Verification items for the finished model (mm, model axes). Coordinates: 2 decimals unless noted, no trailing zeros. Write each loop counter-clockwise with the first axis right and the second up, starting at its lowest first coordinate (ties: lowest second). Pieces come first, ordered by that corner, then holes. Notation, with made-up numbers: M -28,84 L 19,84 A22 ccw 19,102 Z; hole C -38.75,-0.5 d3. An arc over 180 degrees is marked long. Answer in a Markdown table with one row per item.
from build123d import *

# Parameters (mm, degrees)
SKETCH1_W           = 45
SKETCH1_H           = 75
BOSS_EXTRUDE1_DEPTH = 1
SKETCH2_W           = 23
SKETCH2_H           = 16.479286024
BOSS_EXTRUDE2_DEPTH = 1
SKETCH3_W           = 15.006040788
SKETCH3_H           = 6.122008564
BOSS_EXTRUDE3_DEPTH = 1


with BuildPart() as part:
    # Sketch1 → Boss-Extrude1 (new body)
    with BuildSketch(Plane.XY):
        Rectangle(SKETCH1_W, SKETCH1_H)
    extrude(amount=BOSS_EXTRUDE1_DEPTH)

    # Sketch2 → Boss-Extrude2 (add)
    with BuildSketch(Plane.XY.offset(1)):
        with Locations((11, -45.739643012)):
            Rectangle(SKETCH2_W, SKETCH2_H)
    extrude(amount=-BOSS_EXTRUDE2_DEPTH)

    # Sketch3 → Boss-Extrude3 (add)
    with BuildSketch(Plane.XY.offset(1)):
        with Locations((-14.996979606, 40.561004282)):
            Rectangle(SKETCH3_W, SKETCH3_H)
    extrude(amount=-BOSS_EXTRUDE3_DEPTH)


solid = part.part
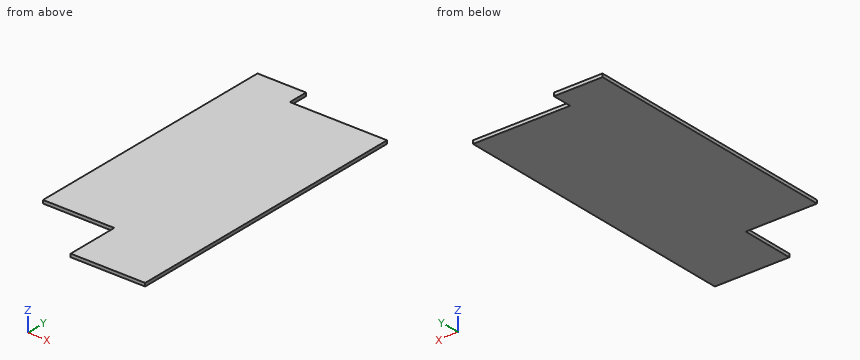
1) Depth check by flat-ended pin: pin 1 (0.5 mm diameter, centred on y = -48, z = 0.5, fed in from -X). Enter the tip coordinate at first touch or a pass-through.
Response values:
| item | result |
|---|---|
| pin 1 | stops at x = -0.5 |
2) Sectioned sample at B-B (x = 3.5). Record the cut outline in (y, z), then the cut area to 3 significant figures.
Response values:
| item | result |
|---|---|
| outline | M -53.98,0 L 37.5,0 L 37.5,1 L -53.98,1 Z |
| area | 91.5 mm² |
3) Sectioned sample at C-C (y = -41). Record the cut outline in (x, z), then the cut area to 3 significant figures.
Response values:
| item | result |
|---|---|
| outline | M -0.5,0 L 22.5,0 L 22.5,1 L -0.5,1 Z |
| area | 23.0 mm² |
4) Sectioned sample at A-A (z = 0.75). Record the cut outline in (x, y).
Response values:
| item | result |
|---|---|
| outline | M -22.5,-37.5 L -0.5,-37.5 L -0.5,-53.98 L 22.5,-53.98 L 22.5,37.5 L -7.49,37.5 L -7.49,43.62 L -22.5,43.62 Z |
5) Thickness scan on L1, parallel to Y at x = 5, z = 0.8; L2, parallel to X at y = -44.5, z = 0.1; L3, parallel to Y at x = -15, z = 0.9. Record the ranges inside material, lowest first. Write a range as [from, to].
Response values:
| item | result |
|---|---|
| L1 | y = [-53.98, 37.5] |
| L2 | x = [-0.5, 22.5] |
| L3 | y = [-37.5, 43.62] |
